Autodesk Inventor part; units mm, degrees
ref_plane "Work Plane1" through (0, 0, -15) normal (0, 0, 1) x (1, 0, 0)
ref_plane "YZ Plane" through (0, 0, 0) normal (1, 0, 0) x (0, 1, 0)
ref_plane "XZ Plane" through (0, 0, 0) normal (0, 1, 0) x (-1, 0, 0)
sketch "Sketch1" plane through (0, 0, 0) normal (0, 0, 1) x (1, 0, 0)
  line L0 (0, 0) -> (25, 0)
  line L1 (25, 0) -> (25, 40)
  line L2 (25, 40) -> (0, 40)
  line L3 (0, 40) -> (0, 0)
  dimension "d1" = 25
  dimension "d2" = 40
  dimension "d3" = 25
extrude "Extrusion1" add sketch "Sketch1" against normal blind 30
sketch "Sketch2" plane through (25, 0, 0) normal (1, 0, 0) x (0, 0, -1)
  line L0 (0, 0) -> (30, 0)
  circle A0 centre (15, 6.56) radius 2.46
extrude "Extrusion2" cut sketch "Sketch2" against normal blind 30
sketch "Sketch3" plane through (0, 0, 0) normal (-1, 0, 0) x (0, 0, 1)
  line L0 (0, 0) -> (-30, 0)
  line L1 (-25.05, 0) -> (-4.95, 0)
  line L2 (-4.95, 0) -> (-4.95, 33.12)
  line L3 (-4.95, 33.12) -> (-25.05, 33.12)
  line L4 (-25.05, 33.12) -> (-25.05, 0)
  dimension "d11" = 20.1
extrude "Extrusion3" cut sketch "Sketch3" against normal blind 20
sketch "Sketch4" plane through (0, 0, 0) normal (0, -1, 0) x (1, 0, 0)
  line L0 (20, -4.95) -> (20, -25.05)
  line L1 (20, -15) -> (25, -15)
  line L2 (25, 0) -> (25, -30)
  line L3 (20, -8.025) -> (25, -8.025)
  line L4 (25, -8.025) -> (25, -21.975)
  line L5 (25, -21.975) -> (20, -21.975)
  line L6 (20, -21.975) -> (20, -8.025)
  line L7 (20, -8.025) -> (25, -21.975) construction
  line L8 (25, -8.025) -> (20, -21.975) construction
  line L9 (25, -12.54) -> (25, -17.46)
  point P0 (0, 0)
  point P1 (22.5, -15)
  dimension "d14" = 13.95
extrude "Extrusion4" add sketch "Sketch4" along normal blind 15
sketch "Sketch5" plane through (20, 0, 0) normal (-1, 0, 0) x (0, 0, 1)
  circle A0 centre (-15, 6.56) radius 2.46
  circle A1 centre (-15, 6.56) radius 4.7025
  circle A2 centre (-15, 6.56) radius 2.46
  circle A3 centre (-15, 6.56) radius 2.46
  point P0 (0, 0)
  dimension "d17" = 9.405
extrude "Extrusion5" cut sketch "Sketch5" against normal blind 2.1
sketch "Sketch6" plane through (25, 0, 0) normal (1, 0, 0) x (0, 0, -1)
  circle A0 centre (15, 6.56) radius 4.7025
  line L0 (15, 6.56) -> (15, 23.56)
  circle A1 centre (15, 23.56) radius 2.46
  point P0 (0, 0)
  dimension "d20" = 17
  dimension "d21" = 4.92
extrude "Extrusion6" cut sketch "Sketch6" against normal blind 10 contours A1
sketch "Sketch7" plane through (20, 0, 0) normal (-1, 0, 0) x (0, 0, 1)
  circle A0 centre (-15, 23.56) radius 2.46
  circle A1 centre (-15, 23.56) radius 4.7025
  point P0 (0, 0)
  dimension "d24" = 9.405
extrude "Extrusion7" cut sketch "Sketch7" against normal blind 2.1
sketch "Sketch9" plane through (25, 0, 0) normal (1, 0, 0) x (0, 0, -1)
  circle A0 centre (15, 6.56) radius 2.46
  circle A1 centre (15, 6.56) radius 2.46
  circle A2 centre (15, 23.56) radius 2.46
  circle A3 centre (15, 23.56) radius 2.46
  line L0 (30, 40) -> (30, 0)
  line L1 (30, 0) -> (30, 40)
  line L2 (30, 40) -> (0, 40)
  line L3 (0, 40) -> (0, 0)
  line L4 (0, 0) -> (8.025, 0)
  line L5 (21.975, 0) -> (21.975, -15)
  line L6 (21.975, -15) -> (8.025, -15)
  line L7 (8.025, -15) -> (8.025, 0)
  line L8 (0, 0) -> (8.025, 0)
  line L9 (21.975, 0) -> (30, 0)
extrude "Extrusion8" add sketch "Sketch9" along normal blind 5
sketch "Sketch10" plane through (0, 40, 0) normal (0, 1, 0) x (1, 0, 0)
  line L0 (0, 30) -> (30, 30)
  line L1 (30, 0) -> (0, 0)
  line L2 (0, 30) -> (30, 30)
  line L3 (30, 30) -> (30, 0)
  line L4 (30, 0) -> (0, 0)
  line L5 (0, 0) -> (0, 30)
extrude "Extrusion9" add sketch "Sketch10" along normal blind 30
sketch "Sketch12" plane through (30, 0, 0) normal (1, 0, 0) x (0, 0, -1)
  circle A0 centre (15, 6.56) radius 2.46
  line L0 (15, 6.56) -> (15, 15.06)
  circle A1 centre (15, 15.06) radius 2.525
  point P0 (0, 0)
  dimension "d31" = 8.5
  dimension "d33" = 5.05
extrude "Extrusion10" cut sketch "Sketch12" against normal blind 30 contours A1
sketch "Sketch14" plane through (0, 0, 0) normal (0, 0, 1) x (1, 0, 0)
  line L0 (30, 70) -> (0, 70)
  line L1 (0, 70) -> (0, 85)
  line L2 (-15, 100) -> (-23, 100)
  line L3 (30, 0) -> (30, 70)
  line L4 (30, 113) -> (30, 70)
  arc A0 (0, 85) -> (-15, 100) centre (-15, 85) ccw
  line L5 (30, 105) -> (30, 100)
  line L6 (-23, 128) -> (15, 128)
  line L7 (30, 113) -> (15, 128)
  line L8 (-23, 128) -> (-23, 100)
  point P0 (0, 0)
  point P1 (0, 100)
  dimension "d47" = 30
  dimension "d54" = 15
  dimension "d69" = 28
extrude "Extrusion12" add sketch "Sketch14" against normal blind 30
sketch "Sketch15" plane through (0, 0, -25.05) normal (-1, 0, 0) x (0, 0, 1)
  line L0 (0, 33.12) -> (20.1, 33.12)
  line L1 (20.1, 33.12) -> (20.1, 0)
  line L2 (0, 33.12) -> (20.1, 33.12)
  line L3 (20.1, 33.12) -> (20.1, 31.1)
  line L4 (20.1, 31.1) -> (0, 31.1)
  line L5 (0, 31.1) -> (0, 33.12)
  point P0 (25.05, 0)
  dimension "d57" = 2.02
extrude "Extrusion13" add sketch "Sketch15" against normal blind 20
sketch "Sketch20" plane through (0, 0, 0) normal (0, 0, 1) x (1, 0, 0)
  arc A0 (0, 85) -> (-15, 100) centre (-15, 85) ccw
  arc A1 (0, 85) -> (-15, 100) centre (-15, 85) ccw
  line L0 (-15, 100) -> (-23, 100)
  line L1 (-15, 100) -> (-23, 100)
  line L2 (-23, 128) -> (15, 128)
  line L3 (-23, 128) -> (15, 128)
  line L4 (15, 128) -> (30, 113)
  line L5 (15, 128) -> (30, 113)
  line L6 (30, 113) -> (30, 85)
  line L7 (30, 0) -> (30, 113)
  line L8 (30, 85) -> (0, 85)
  line L9 (-23, 128) -> (-23, 100)
  point P0 (0, 0)
  point P1 (-19, 102)
  point P2 (-15, 114)
  point P3 (-19, 126)
extrude "Extrusion14" add sketch "Sketch20" along normal blind 15
ref_plane "Work Plane1" through (0, 0, -15) normal (0, 0, 1) x (1, 0, 0)
mirror "Mirror1" about plane through (0, 0, -15) normal (0, 0, 1) of "Extrusion14"
sketch "Sketch21" plane through (-23, 128, 15) normal (0, 1, 0) x (1, 0, 0)
  line L0 (0, 0) -> (0, 60)
  line L1 (0, 30) -> (0, 12.5)
  line L2 (0, 47.5) -> (0, 30)
  line L3 (0, 47.5) -> (10, 30)
  line L4 (10, 30) -> (0, 12.5)
  point P0 (23, 15)
  dimension "d76" = 17.5
extrude "Extrusion15" cut sketch "Sketch21" against normal through all
properties part number "24mm_x_60mm"
Geometry: final body of the model. Coordinates: model frame, mm. A direction names the side the tool comes from. Round coordinates to 2 decimals unless told otherwise and drop trailing zeros. Write each loop counter-clockwise with the first axis right and the second up, starting at its lowest first coordinate (ties: lowest second). Pieces come first, ordered by that corner, then holes.
Item 1: Material intervals for L1, parallel to Y at x = 21.4, z = -15 (1 decimal); L2, parallel to Z at x = 25.25, y = 15.06 (3 decimals); L3, parallel to Y at x = 13, z = -28, sorted ascending.
Item 2: Section query C-C (y = 111). Return loops of the section in (x, z).
Item 3: Section query D-D (x = -5.5). Return loops of the section in (y, z).
Item 4: Section query B-B (z = -38). Return loops of the section in (x, y).
Item 5: Pin query (flat end, axial travel): P1, Ø1.5, axis at x = -12.5, z = -12.5, coming from the -Y side; P2, Ø4.5, axis at y = 22, z = -17, coming from the -X side; P3, Ø11, axis at x = 23, y = -4.5, coming from the +Z side. Return the tip coordinate at first contact, or that it passes through.
Item 6: Mould query, pull axis Y, two halves, no side actions, for faces 1 (the face through (3, 107, 15)), 2 (the face through (25.995, 24.502, -17.272)), 3 (the face through (18, 0, -27)). Classes: +Y half, -Y half, draft (parallel to the pull), parting line (faces both ways), or undercut.
Item 7: Set-up query: faces 4 (the face through (-18, 100, -35)), 5 (the face through (22.1, 21.5, -13)), 6 (the face through (20, 8, -20)), 7 (the face through (25, -7, -21.975)), 8 (the face through (15, 0, -3)). Return all of +Z, -Z, +X, -X, +Y, -Y with unobstructed straight access to the full face (end or side cutting, diameter ignored); none if empty.
Item 8: Section query A-A (y = 15.06). Return loops of the section in (x, z) (3 decimals).
Completed:
1. L1: y = -15 to 1.9, 11.3 to 12.5, 17.6 to 18.9, 28.3 to 121.6
1. L2: z = -30 to -17.525, -12.475 to 0
1. L3: y = 0 to 128
2. outline: (-23, -45) - (30, -45) - (30, 15) - (-23, 15) - (-23, 2.5) - (-13, -15) - (-23, -32.5) - close
3. outline: (96.61, -45) - (128, -45) - (128, 15) - (96.61, 15) - close
4. outline: (-23, 100) - (-15, 100) arc R15 cw to (0, 85) - (30, 85) - (30, 113) - (15, 128) - (-23, 128) - close
5. P1: stops at y = 99.64
5. P2: stops at x = 20
5. P3: stops at z = 0
6. face 1: draft
6. face 2: undercut
6. face 3: -Y half
7. face 4: +Z, -Z, -X, -Y
7. face 5: -X
7. face 6: -X, -Y
7. face 7: -Z, +X, -X, -Y
7. face 8: +Z, +X, -X, -Y
8. outline: (0, -30) - (30, -30) - (30, -17.525) - (20, -17.525) - (20, -25.05) - (0, -25.05) - close; (0, -4.95) - (20, -4.95) - (20, -12.475) - (30, -12.475) - (30, 0) - (0, 0) - close
